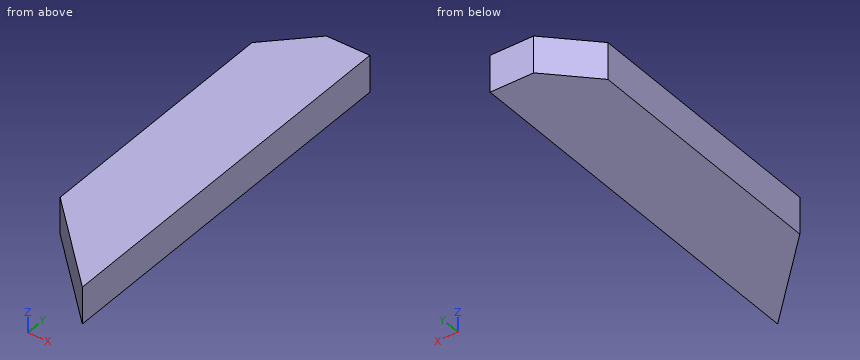
```python
from build123d import *

# Parameters (mm, degrees)
SKETCH1_W           = 88.9
SKETCH1_H           = 38.1
BOSS_EXTRUDE1_DEPTH = 444.5
CUT_EXTRUDE1_DEPTH  = 449.338780946
CUT_EXTRUDE2_DEPTH  = 449.338780946


with BuildPart() as part:
    # Sketch1 → Boss-Extrude1 (new body)
    with BuildSketch(Plane(origin=(0, 0, 0), x_dir=(1, 0, 0), z_dir=(0, 1, 0))):
        Rectangle(SKETCH1_W, SKETCH1_H)
    extrude(amount=BOSS_EXTRUDE1_DEPTH)

    # Sketch2 → Cut-Extrude1 (cut, through all)
    with BuildSketch(Plane.XY.offset(19.05)):
        Polygon((-44.45, 444.5), (44.45, 444.5), (-44.45, 355.6), align=None)
        Polygon((44.45, 0), (-44.45, 0), (-44.45, 88.9), align=None)
    extrude(amount=-CUT_EXTRUDE1_DEPTH, mode=Mode.SUBTRACT)

    # Sketch3 → Cut-Extrude2 (cut, through all)
    with BuildSketch(Plane.XY.offset(19.05)):
        Polygon((44.45, 444.5), (-0.451280605, 399.598719395), (44.45, 399.598719395), align=None)
    extrude(amount=-CUT_EXTRUDE2_DEPTH, mode=Mode.SUBTRACT)


solid = part.part
```
Input: part model. Units: mm. Frame: model coordinates. Coordinates: 2 decimals unless noted, no trailing zeros. Write each loop counter-clockwise with the first axis right and the second up, starting at its lowest first coordinate (ties: lowest second). Pieces come first, ordered by that corner, then holes.
1) Section B-B on x = -22.5. Output: boundary loops of the cut face in (y, z), and give its area (3 significant figures).
2) Section C-C on y = 372. Output: boundary loops of the cut face in (x, z).
3) Pin query (flat end, axial travel): pin 1 Ø1.5 at (x, z) = (-12.5, -1) entering from +Y; pin 2 Ø5 at (x, z) = (-5.5, -5.5) entering from +Y; pin 3 Ø10 at (y, z) = (44.5, 6.5) entering from -X. Return the tip coordinate at first contact, or that it passes through.
4) Material intervals for line 1 along Y through (x, z) = (12.5, -14); line 2 along Y through (x, z) = (6.5, -16.5); line 3 along X through (y, z) = (77, 4.5), sorted ascending.
5) Section A-A on z = 6. Output: boundary loops of the cut face in (x, y).
Check result:
1. outline: (66.95, -19.05) - (377.55, -19.05) - (377.55, 19.05) - (66.95, 19.05) - close
1. area: 11,800 mm2
2. outline: (-28.05, -19.05) - (44.45, -19.05) - (44.45, 19.05) - (-28.05, 19.05) - close
3. pin 1: stops at y = 388.3
3. pin 2: stops at y = 397.05
3. pin 3: stops at x = -5.05
4. line 1: y = 31.95 to 399.6
4. line 2: y = 37.95 to 399.6
4. line 3: x = -32.55 to 44.45
5. outline: (-44.45, 88.9) - (44.45, 0) - (44.45, 399.6) - (-0.45, 399.6) - (-44.45, 355.6) - close
